from build123d import *

# Parameters (mm, degrees)
F0_W     = 88.9
F0_H     = 50.8
F1_DEPTH = 34.925
F2_R     = 3.175
F3_DEPTH = 34.925


with BuildPart() as f1:
    # F0 (on Front) → F1 (new body)
    with BuildSketch(Plane.XZ):
        with Locations((-50.103806, 54.703811)):
            Rectangle(F0_W, F0_H)
    extrude(amount=F1_DEPTH)

    # F2 (on face) → F3 (cut)
    with BuildSketch(Plane.XZ.offset(34.925)):
        with Locations((-81.853806, 67.403811)):
            Circle(F2_R)
        with Locations((-81.853806, 35.653811)):
            Circle(F2_R)
        with Locations((-18.353806, 67.403811)):
            Circle(F2_R)
        with Locations((-18.353806, 35.653811)):
            Circle(F2_R)
    extrude(amount=-F3_DEPTH, mode=Mode.SUBTRACT)


solid = f1.part
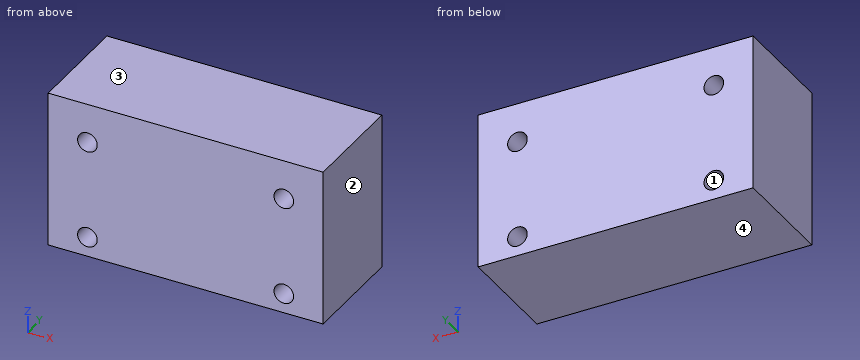
Model file for the job. Use its own axes, mm. Face numbers are marked on the shaded views. Round coordinates to 2 decimals unless told otherwise and drop trailing zeros. Loops run counter-clockwise (first coordinate to the right, second up) from the corner with the lowest first, then second, coordinate; pieces in that order, holes last. Notation, with made-up numbers: (38.25, 10) - (59.25, 10) arc R34 cw to (59.25, 45) - close; hole circle Ø6 at (-29, 16.5). An arc over 180 degrees is marked (long way). Write each question's results on one line, items separated by ' | '.
(1) Mould opens along Z. For the marked faces 1, 2, 3 and 4 say: released by +Z, released by -Z, zero draft, split by the parting line, or undercut.
Answer below:
face 1: undercut | face 2: zero draft | face 3: released by +Z | face 4: released by -Z
(2) Pin check, flat tips, straight feed: pin 1 (2 mm diameter, centred on x = -47.5, z = 60, fed in from +Y); pin 2 (4 mm diameter, centred on x = -18.35, z = 67.4, fed in from -Y). Stop position of each tip, or through.
Answer below:
pin 1: stops at y = 0 | pin 2: passes through
(3) Saw through at A-A, the plane z = 66. List the corners of the cut face in (x, y) (3 decimals).
Answer below:
outline: (-94.554, -34.925) - (-84.702, -34.925) - (-84.702, 0) - (-94.554, 0) - close; (-79.006, -34.925) - (-21.202, -34.925) - (-21.202, 0) - (-79.006, 0) - close; (-15.506, -34.925) - (-5.654, -34.925) - (-5.654, 0) - (-15.506, 0) - close
(4) Wall check: L1, parallel to X at y = -19.5, z = 68.5; L2, parallel to X at y = -30.5, z = 69; L3, parallel to Z at x = -84, y = -20. Give the ranges that are in metal, low to high.
Answer below:
L1: x = -94.55 to -84.83, -78.87 to -21.33, -15.37 to -5.65 | L2: x = -94.55 to -84.6, -79.11 to -21.1, -15.61 to -5.65 | L3: z = 29.3 to 33.31, 37.99 to 65.06, 69.74 to 80.1
(5) Saw through at B-B, the plane y = -5. List the corners of the cut face in (x, z) (3 decimals), then the cut area to 3 significant figures.
Answer below:
outline: (-94.554, 29.304) - (-5.654, 29.304) - (-5.654, 80.104) - (-94.554, 80.104) - close; hole circle Ø6.35 at (-81.854, 35.654); hole circle Ø6.35 at (-81.854, 67.404); hole circle Ø6.35 at (-18.354, 35.654); hole circle Ø6.35 at (-18.354, 67.404) | area: 4,390 mm^2
